Here's how the part is built. I have some questions about the finished solid (model axes, mm). Give positions to 0.01 mm unless a question says otherwise; leave off trailing zeros. Loops run counter-clockwise (first coordinate to the right, second up) from the corner with the lowest first, then second, coordinate; pieces in that order, holes last. Notation, with made-up numbers: (37.25, 62) - (67.25, 62) arc R25 cw to (67.25, 87) - close; hole circle Ø7 at (17, 40). An arc over 180 degrees is marked (long way). Return JSON: item names as keys, results as strings. Group by question number.
(1) If we section it at D-D (z = 19.05): Please give me the cut outline in (x, y), then the cut area to 3 significant figures.
(2) If we section it at A-A (z = 57.15): Please give me the cut outline in (x, y), then the cut area to 3 significant figures.
(3) If we section it at B-B (y = 11.25): State how many separate pieces and enclosed holes the cut face has, then the cut area to 3 significant figures.
(4) If we section it at C-C (x = -31.75): Please give me the cut outline in (y, z).
(5) If we mould it in two halves opening along Z, with no side actions, what happens to faces 1 (the flat face through (-1, 6, -63.5)), 2 (the cylindrical face through (27.207, 6.261, -33.181)), 3 (the flat face through (-50.8, 6, 1)), 4 (the cylindrical face through (-29.392, 7.406, 58.128))? For each: released by +Z, released by -Z, zero draft, split by the parting line, or undercut.
(6) I need wall thicknesses on probe 1 along X at (y, z) = (7.75, 19.05); probe 2 along Z at (x, y) = (31.75, 8); probe 3 along Z at (x, y) = (35, 12.25). Which ranges of each line are inside material? Lowest first, please. Write a range as [from, to].
```python
from build123d import *

# Parameters (mm, degrees)
SKETCH1_W                                          = 101.6
SKETCH1_H                                          = 127
BOSS_EXTRUDE1_DEPTH                                = 12.7
CSK_FOR_10_FLAT_HEAD_MACHINE_SCREW_100_D           = 5.1054
CSK_FOR_10_FLAT_HEAD_MACHINE_SCREW_100_DEPTH       = 12.7
CSK_FOR_10_FLAT_HEAD_MACHINE_SCREW_100_CSINK_D     = 9.779
CSK_FOR_10_FLAT_HEAD_MACHINE_SCREW_100_CSINK_ANGLE = 100
CSK_FOR_10_FLAT_HEAD_MACHINE_SCREW_100_TIP         = 1.533816902
F_3_8_0_375_DIAMETER_HOLE1_D                       = 9.525
F_3_8_0_375_DIAMETER_HOLE1_DEPTH                   = 25.4
F_3_8_0_375_DIAMETER_HOLE1_TIP                     = 2.861598698


with BuildPart() as part:
    # Sketch1 → Boss-Extrude1 (new body)
    with BuildSketch(Plane(origin=(0, 0, 0), x_dir=(1, 0, 0), z_dir=(0, 1, 0))):
        Rectangle(SKETCH1_W, SKETCH1_H)
    extrude(amount=BOSS_EXTRUDE1_DEPTH)

    # CSK for #10 Flat Head Machine Screw (100)1
    with Locations(Plane(origin=(0, 0, 0), x_dir=(-1, 0, 0), z_dir=(0, -1, 0))):
        with Locations((31.75, -57.15), (-31.75, -57.15)):
            CounterSinkHole(CSK_FOR_10_FLAT_HEAD_MACHINE_SCREW_100_D / 2, CSK_FOR_10_FLAT_HEAD_MACHINE_SCREW_100_CSINK_D / 2, depth=CSK_FOR_10_FLAT_HEAD_MACHINE_SCREW_100_DEPTH, counter_sink_angle=CSK_FOR_10_FLAT_HEAD_MACHINE_SCREW_100_CSINK_ANGLE)
            with Locations((0, 0, -(CSK_FOR_10_FLAT_HEAD_MACHINE_SCREW_100_DEPTH + CSK_FOR_10_FLAT_HEAD_MACHINE_SCREW_100_TIP / 2))):  # 118° drill point
                Cone(0, CSK_FOR_10_FLAT_HEAD_MACHINE_SCREW_100_D / 2, CSK_FOR_10_FLAT_HEAD_MACHINE_SCREW_100_TIP, mode=Mode.SUBTRACT)

    # 3/8 (0.375) Diameter Hole1
    with Locations(Plane(origin=(0, 12.7, 0), x_dir=(1, 0, 0), z_dir=(0, 1, 0))):
        with Locations((-31.75, 31.75), (31.75, 31.75), (-31.75, -19.05), (31.75, -19.05)):
            Hole(F_3_8_0_375_DIAMETER_HOLE1_D / 2, depth=F_3_8_0_375_DIAMETER_HOLE1_DEPTH)
            with Locations((0, 0, -(F_3_8_0_375_DIAMETER_HOLE1_DEPTH + F_3_8_0_375_DIAMETER_HOLE1_TIP / 2))):  # 118° drill point
                Cone(0, F_3_8_0_375_DIAMETER_HOLE1_D / 2, F_3_8_0_375_DIAMETER_HOLE1_TIP, mode=Mode.SUBTRACT)


solid = part.part
```
Values:
{
 "1": {"outline": "(-50.8, 0) - (-36.51, 0) - (-36.51, 12.7) - (-50.8, 12.7) - close; (-26.99, 0) - (26.99, 0) - (26.99, 12.7) - (-26.99, 12.7) - close; (36.51, 0) - (50.8, 0) - (50.8, 12.7) - (36.51, 12.7) - close", "area": "1,050 mm2"},
 "2": {"outline": "(-50.8, 0) - (-36.64, 0) - (-34.3, 1.96) - (-34.3, 12.7) - (-50.8, 12.7) - close; (-29.2, 1.96) - (-26.86, 0) - (26.86, 0) - (29.2, 1.96) - (29.2, 12.7) - (-29.2, 12.7) - close; (34.3, 1.96) - (36.64, 0) - (50.8, 0) - (50.8, 12.7) - (34.3, 12.7) - close", "area": "1,150 mm2"},
 "3": {"separate pieces": "1", "enclosed holes": "6", "area": "12,600 mm2"},
 "4": {"outline": "(0, -63.5) - (12.7, -63.5) - (12.7, -36.51) - (0, -36.51) - close; (0, -26.99) - (12.7, -26.99) - (12.7, 14.29) - (0, 14.29) - close; (0, 23.81) - (12.7, 23.81) - (12.7, 54.6) - (1.96, 54.6) - (0, 52.26) - close; (0, 62.04) - (1.96, 59.7) - (12.7, 59.7) - (12.7, 63.5) - (0, 63.5) - close"},
 "5": {"face 1": "released by -Z", "face 2": "undercut", "face 3": "zero draft", "face 4": "undercut"},
 "6": {"probe 1": "[-50.8, -36.51], [-26.99, 26.99], [36.51, 50.8]", "probe 2": "[-63.5, -36.51], [-26.99, 14.29], [23.81, 54.6], [59.7, 63.5]", "probe 3": "[-63.5, -35.23], [-28.27, 15.57], [22.53, 63.5]"}
}
